Could you check a few things on this model? Use its own coordinates, in mm. A direction names the side the tool comes from. Give positions to 0.01 mm unless a question says otherwise; leave off trailing zeros. Order: outer loops, then holes, each group sorted by start corner. A loop starts at its lowest first (then second) coordinate and runs counter-clockwise, first axis right, second up.
from build123d import *

# Parameters (mm, degrees)
F0_R     = 3.2
F1_DEPTH = 10
F2_R     = 3.2
F3_DEPTH = 5
F4_SIZE  = 1


with BuildPart() as f1:
    # F0 (on Top) → F1 (new body)
    with BuildSketch(Plane.XY):
        Circle(F0_R)
    extrude(amount=F1_DEPTH)

    # F2 (on face) → F3 (join)
    with BuildSketch(Plane.XY.offset(10)):
        Polygon((3.75, -6.495191), (7.5, 0), (3.75, 6.495191), (-3.75, 6.495191), (-7.5, 0), (-3.75, -6.495191), align=None)
        Circle(F2_R, mode=Mode.SUBTRACT)
        Circle(F2_R)
    extrude(amount=F3_DEPTH)

    # F4
    f4_edges = [f1.edges().sort_by_distance(p)[0] for p in [
        (0, -6.495191, 15),
        (5.625, -3.247595, 15),
        (5.625, 3.247595, 15),
        (0, 6.495191, 15),
        (-5.625, 3.247595, 15),
        (-5.625, -3.247595, 15),
        (-3.2, 0, 0),
    ]]
    chamfer(f4_edges, length=F4_SIZE)


solid = f1.part
Item 1: Please list where these lines run through material, in increasing order: line 1 along Z through (x, y) = (-3, 5.25); line 2 along Y through (x, z) = (0, 4); line 3 along X through (y, z) = (1.5, 14.75).
Findings:
line 1: z = 10 to 15
line 2: y = -3.2 to 3.2
line 3: x = -5.77 to 5.77
Item 2: Imagine slicing it at A-A on x = 0. List the corners of the cut face in (y, z) for me, then the cut area to 3 significant figures.
Findings:
outline: (-6.5, 10) - (-3.2, 10) - (-3.2, 1) - (-2.2, 0) - (2.2, 0) - (3.2, 1) - (3.2, 10) - (6.5, 10) - (6.5, 14) - (5.5, 15) - (-5.5, 15) - (-6.5, 14) - close
area: 127 mm2
Item 3: Imagine slicing it at D-D on z = 2.5. List the corners of the cut face in (x, y) for me, then the cut area to 3 significant figures.
Findings:
outline: circle Ø6.4 at (0, 0)
area: 32.2 mm2
Item 4: For faces 1 (the flat face through (-5.651, -3.202, 11.972)), 2 (the flat face through (2, 3, 10)), which set-ups out of +Z, -Z, +X, -X, +Y, -Y let a thin tool reach every point of the face, with its end or its side?
Findings:
face 1: +Z, -Z, -X, -Y
face 2: -Z
Item 5: Imagine slicing it at C-C on y = -4.25. List the corners of the cut face in (x, z) for me, then the cut area to 3 significant figures.
Findings:
outline: (-5.05, 10) - (5.05, 10) - (5.05, 14) - (3.89, 15) - (-3.89, 15) - (-5.05, 14) - close
area: 49.3 mm2
Item 6: Imagine slicing it at B-B on z = 11.5. List the corners of the cut face in (x, y) for me.
Findings:
outline: (-7.5, 0) - (-3.75, -6.5) - (3.75, -6.5) - (7.5, 0) - (3.75, 6.5) - (-3.75, 6.5) - close
Item 7: For pin 1 (1.5 mm diameter, centred on y = -2.5, z = 8, fed in from -X); pin 2 (3 mm diameter, centred on y = -2, z = 3, fed in from +X); pin 3 (2 mm diameter, centred on y = -2, z = 5.5, fed in from +X), each with a flat end and sliding along its axis, tell me the tip position at first contact or that it passes through.
Findings:
pin 1: stops at x = -2.68
pin 2: stops at x = 3.16
pin 3: stops at x = 3.04
